Geometry check sheet. Reference: the model listing, model coordinates, mm. Face numbers are marked on the shaded views. Give positions to 0.01 mm unless a question says otherwise; leave off trailing zeros. Write each loop counter-clockwise with the first axis right and the second up, starting at its lowest first coordinate (ties: lowest second). Pieces come first, ordered by that corner, then holes. Notation, with made-up numbers: (12.5, 44.25) -> (70.5, 44.25) arc R17 ccw to (70.5, 65.25) -> close; hole circle Ø5 at (6.25, -36). An arc over 180 degrees is marked (long way). Use a Markdown table: item, result. Add a question column.
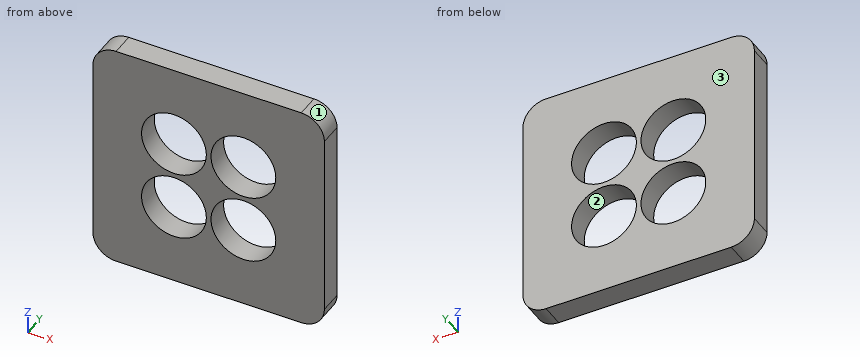
from build123d import *

# Parameters (mm, degrees)
F1_DEPTH = 5
F2_R     = 7
F3_DEPTH = 5.001


with BuildPart() as f1:
    # F0 (on Front) → F1 (new body)
    with BuildSketch(Plane.XZ):
        with BuildLine():
            Line((-5, 50), (-45, 50))
            ThreePointArc((-45, 50), (-48.535534, 48.535534), (-50, 45))
            Line((-50, 45), (-50, 5))
            ThreePointArc((-50, 5), (-48.535534, 1.464466), (-45, 0))
            Line((-45, 0), (-5, 0))
            ThreePointArc((-5, 0), (-1.464466, 1.464466), (0, 5))
            Line((0, 5), (0, 45))
            ThreePointArc((0, 45), (-1.464466, 48.535534), (-5, 50))
        make_face()
    extrude(amount=F1_DEPTH)

    # F2 (on face) → F3 (cut, through all)
    with BuildSketch(Plane.XZ.offset(5)):
        with Locations((-17.5, 32.5)):
            Circle(F2_R)
        with Locations((-32.5, 32.5)):
            Circle(F2_R)
        with Locations((-17.5, 17.5)):
            Circle(F2_R)
        with Locations((-32.5, 17.5)):
            Circle(F2_R)
    extrude(amount=-F3_DEPTH, mode=Mode.SUBTRACT)


solid = f1.part
1) Draft check along Z on the marked faces 1, 2 and 3. Enter one of: +Z half, -Z half, draft (parallel to the pull), parting line (faces both ways), or undercut.
2) Sectioned sample at C-C, the plane x = -17.5. Enter the section's corners in (y, z), and give its area (3 significant figures).
3) Sectioned sample at B-B, the plane y = -2.5. Enter the section's corners in (x, z).
4) Sectioned sample at A-A, the plane z = 17.5. Enter the section's corners in (x, y).
5) Material ranges on probe 1 along Z at (x, y) = (-17.5, -2.8); probe 2 along X at (y, z) = (-1.2, 37.5); probe 3 along Z at (x, y) = (-23, -4.6), recorded low to high. Write a range as [from, to].
6) Gauge pin test, flat end, axial feed: P1, Ø6, axis at x = -30, z = 32, coming from the +Y side. Record the tip position at first contact, or that the pin passes through.
Check values:
| question | item | result |
|---|---|---|
| 1 | face 1 | +Z half |
| 1 | face 2 | undercut |
| 1 | face 3 | draft |
| 2 | outline | (-5, 0) -> (0, 0) -> (0, 10.5) -> (-5, 10.5) -> close; (-5, 24.5) -> (0, 24.5) -> (0, 25.5) -> (-5, 25.5) -> close; (-5, 39.5) -> (0, 39.5) -> (0, 50) -> (-5, 50) -> close |
| 2 | area | 110 mm² |
| 3 | outline | (-50, 5) arc R5 ccw to (-45, 0) -> (-5, 0) arc R5 ccw to (0, 5) -> (0, 45) arc R5 ccw to (-5, 50) -> (-45, 50) arc R5 ccw to (-50, 45) -> close; hole circle Ø14 at (-32.5, 17.5); hole circle Ø14 at (-32.5, 32.5); hole circle Ø14 at (-17.5, 17.5); hole circle Ø14 at (-17.5, 32.5) |
| 4 | outline | (-50, -5) -> (-39.5, -5) -> (-39.5, 0) -> (-50, 0) -> close; (-25.5, -5) -> (-24.5, -5) -> (-24.5, 0) -> (-25.5, 0) -> close; (-10.5, -5) -> (0, -5) -> (0, 0) -> (-10.5, 0) -> close |
| 5 | probe 1 | [0, 10.5], [24.5, 25.5], [39.5, 50] |
| 5 | probe 2 | [-50, -37.4], [-27.6, -22.4], [-12.6, 0] |
| 5 | probe 3 | [0, 13.17], [21.83, 28.17], [36.83, 50] |
| 6 | P1 | through |
